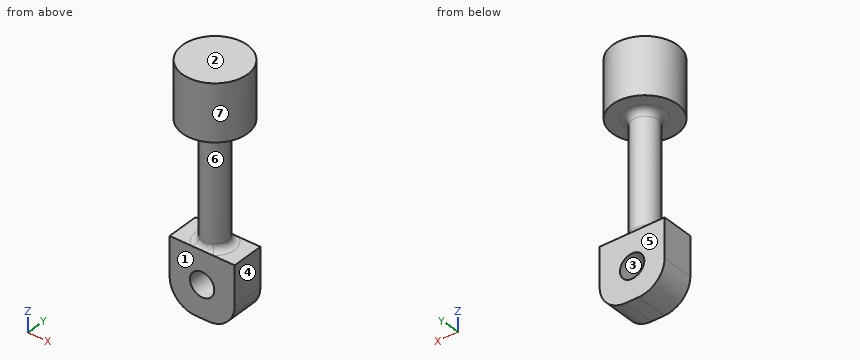
```python
from build123d import *

# Parameters (mm, degrees)
SKETCH1_W                = 1
SKETCH1_H                = 9
SKETCH1_3_R              = 0.935
BOSS_EXTRUDE1_DEPTH      = 1.25
BOSS_EXTRUDE1_DEPTH_BACK = 1.25
FILLET1_R                = 0.5
FILLET2_R                = 0.5


with BuildPart() as part:
    # Sketch1 → Revolve1 (revolve)
    with BuildSketch(Plane(origin=(0, 0, 0), x_dir=(1, 0, 0), z_dir=(0, 1, 0))):
        with Locations((3, -4.5)):
            Rectangle(SKETCH1_W, SKETCH1_H)
    revolve(axis=Axis((2.5, 0, 0), (0, 0, -1)))

    # Sketch1_3 → Boss-Extrude1 (add, two sides)
    with BuildSketch(Plane(origin=(0, 0, 0), x_dir=(1, 0, 0), z_dir=(0, 1, 0))) as boss_extrude1_sk:
        with BuildLine():
            Line((0, 0), (5, 0))
            Line((5, 0), (5, 3))
            ThreePointArc((5, 3), (4.414213562, 4.414213562), (3, 5))
            Line((3, 5), (2, 5))
            ThreePointArc((2, 5), (0.585786438, 4.414213562), (0, 3))
            Line((0, 3), (0, 0))
        make_face()
        with Locations((2.5, 2.5)):
            Circle(SKETCH1_3_R, mode=Mode.SUBTRACT)
    extrude(amount=BOSS_EXTRUDE1_DEPTH)
    extrude(boss_extrude1_sk.sketch, amount=-BOSS_EXTRUDE1_DEPTH_BACK)

    # Fillet1
    fillet1_edges = [part.edges().sort_by_distance(p)[0] for p in [
        (1.5, 0, 0),
    ]]
    fillet(fillet1_edges, radius=FILLET1_R)

    # Sketch1_4 → Revolve2 (revolve)
    with BuildSketch(Plane(origin=(0, 0, 0), x_dir=(1, 0, 0), z_dir=(0, 1, 0))):
        Polygon((3.5, -9), (2.5, -9), (2.5, -13.35), (5, -13.35), (5, -9), align=None)
    revolve(axis=Axis((2.5, 0, 0), (0, 0, -1)))

    # Fillet2
    fillet2_edges = [part.edges().sort_by_distance(p)[0] for p in [
        (1.5, 0, 9),
    ]]
    fillet(fillet2_edges, radius=FILLET2_R)


solid = part.part
```
The listing builds one solid part. Answer for the finished solid, in the listing's coordinates (mm). Face numbers are marked on the shaded views. A direction names the side the tool comes from. Give positions to 0.01 mm unless a question says otherwise; leave off trailing zeros. Loops run counter-clockwise (first coordinate to the right, second up) from the corner with the lowest first, then second, coordinate; pieces in that order, holes last. Notation, with made-up numbers: (46.25, 51.25) - (97.25, 51.25) arc R12 cw to (97.25, 64.25) - close; hole circle Ø9 at (-29, 70). An arc over 180 degrees is marked (long way). Return JSON: item names as keys, results as strings. Group by question number.
1. Determine the mould class of the marked faces 1, 2 and 3 for opening direction Z: pulls with the +Z half, pulls with the -Z half, needs draft (parallel to the pull), parting line crosses it, or undercut.
2. Find section B-B (z = -2.5). Write down the section's boundary in (x, y) (3 decimals), then the cut area to 4 significant figures.
3. Straight lines are drawn through the part: line 1 (Z direction, x = 2.5, y = -0.35) (3 decimals); line 2 (X direction, y = 0.35, z = -2.5) (3 decimals); line 3 (Z direction, x = 1.8, y = 1). For each, find the intervals that lie inside material, in ascending order. Write a range as [from, to].
4. Find section C-C (z = 5.75). Write down the section's boundary in (x, y), then the cut area to 3 significant figures.
5. Find section D-D (y = -1.8). Write down the section's boundary in (x, z).
6. Given pin 1 Ø1.5 at (x, z) = (3, -2) entering from +Y; pin 2 Ø1 at (x, z) = (4.5, 9.5) entering from -Y; pin 3 Ø1.5 at (x, z) = (2.5, -2.5) entering from +Y; pin 4 Ø1.5 at (x, z) = (3, -1.5) entering from -Y, each flat-ended and moving along its own axis, determine where each tip first touches the part or whether it passes through.
7. Which of the six approach directions +Z, -Z, +X, -X, +Y, -Y give full straight-line access (tool end or side, diameter ignored) to the marked faces 4, 5, 6 and 7?
8. Find section A-A (y = 0). Write down the section's boundary in (x, z) (3 decimals), then the cut area to 3 significant figures.
Verdict:
{
 "1": {"face 1": "needs draft", "face 2": "pulls with the +Z half", "face 3": "undercut"},
 "2": {"outline": "(0, -1.25) - (1.565, -1.25) - (1.565, 1.25) - (0, 1.25) - close; (3.435, -1.25) - (5, -1.25) - (5, 1.25) - (3.435, 1.25) - close", "area": "7.825 mm^2"},
 "3": {"line 1": "z = [-5, -3.435], [-1.565, 13.35]", "line 2": "x = [0, 1.565], [3.435, 5]", "line 3": "z = [-4.99, -3.12], [-1.88, 0.09], [8.91, 13.35]"},
 "4": {"outline": "circle Ø2 at (2.5, 0)", "area": "3.14 mm^2"},
 "5": {"outline": "(0.77, 9) - (4.23, 9) - (4.23, 13.35) - (0.77, 13.35) - close"},
 "6": {"pin 1": "stops at y = 1.25", "pin 2": "stops at y = -2", "pin 3": "passes through", "pin 4": "stops at y = -1.25"},
 "7": {"face 4": "+Z, -Z, +X, +Y, -Y", "face 5": "-Z, +X, -X, +Y", "face 6": "none", "face 7": "+Z"},
 "8": {"outline": "(0, -3) arc R2 ccw to (2, -5) - (3, -5) arc R2 ccw to (5, -3) - (5, 0) - (4, 0) arc R0.5 cw to (3.5, 0.5) - (3.5, 8.5) arc R0.5 cw to (4, 9) - (5, 9) - (5, 13.35) - (0, 13.35) - (0, 9) - (1, 9) arc R0.5 cw to (1.5, 8.5) - (1.5, 0.5) arc R0.5 cw to (1, 0) - (0, 0) - close; hole circle Ø1.87 at (2.5, -2.5)", "area": "60.5 mm^2"}
}
